Can you work these out from the model? Positions are in its coordinate system, mm. A direction names the side the tool comes from. Round coordinates to 2 decimals unless told otherwise and drop trailing zeros. Loops run counter-clockwise (first coordinate to the right, second up) from the corner with the lowest first, then second, coordinate; pieces in that order, holes last. Notation, with made-up numbers: (50, 14.5) -> (91, 14.5) arc R25 ccw to (91, 27.5) -> close; hole circle Ø4 at (-31.75, 43). An arc over 180 degrees is marked (long way). Use a Markdown table: item, result.
from build123d import *

# Parameters (mm, degrees)
F0_R     = 6
F1_DEPTH = 10


with BuildPart() as f1:
    # F0 (on Top) → F1 (new body)
    with BuildSketch(Plane.XY):
        with BuildLine():
            Line((58.85537, -68.397695), (17.674352, 9.360411))
            ThreePointArc((17.674352, 9.360411), (-7.229789, 18.647524), (-19.364917, -5))
            Line((-19.364917, -5), (0, -80))
            Line((0, -80), (25, -80))
            Line((25, -80), (25, -130))
            Line((25, -130), (56.798395, -90.252006))
            ThreePointArc((56.798395, -90.252006), (61.093013, -79.632266), (58.85537, -68.397695))
        make_face()
        Circle(F0_R, mode=Mode.SUBTRACT)
    extrude(amount=F1_DEPTH)


solid = f1.part
1. I need wall thicknesses on line 1 (X direction, y = -1, z = 2.25); line 2 (X direction, y = -103.5, z = 3); line 3 (X direction, y = -47, z = 0.75). Which ranges of each line are inside material? Lowest first, please.
Answer sheet:
| item | result |
|---|---|
| line 1 | x = -19.97 to -5.92, 5.92 to 23.16 |
| line 2 | x = 25 to 46.2 |
| line 3 | x = -8.52 to 47.52 |
2. I want a section at C-C (x = 39.5). Please give me the cut outline in (y, z) (3 decimals).
Answer sheet:
| item | result |
|---|---|
| outline | (-111.875, 0) -> (-31.851, 0) -> (-31.851, 10) -> (-111.875, 10) -> close |
3. I want a section at D-D (y = -86). Please give me the cut outline in (x, z).
Answer sheet:
| item | result |
|---|---|
| outline | (25, 0) -> (59.4, 0) -> (59.4, 10) -> (25, 10) -> close |
4. If we mould it in two halves opening along X, with no side actions, what happens to faces 1 (the flat face through (12, -80, 5)), 2 (the cylindrical face through (-6, 0, 5)), 3 (the cylindrical face through (61.077, -79.794, 4.93))? For each: +X half, -X half, draft (parallel to the pull), parting line (faces both ways), or undercut.
Answer sheet:
| item | result |
|---|---|
| face 1 | draft |
| face 2 | undercut |
| face 3 | +X half |
5. I want a section at A-A (z = 4). Please give me the cut outline in (x, y), plus the area to 3 significant figures.
Answer sheet:
| item | result |
|---|---|
| outline | (-19.36, -5) -> (0, -80) -> (25, -80) -> (25, -130) -> (56.8, -90.25) arc R20 ccw to (58.86, -68.4) -> (17.67, 9.36) arc R20 ccw to start; hole circle Ø12 at (0, 0) |
| area | 5,820 mm² |
6. Which directions (+Z, -Z, +X, -X, +Y, -Y) give clear straight access to the entire face, cutting with the end or side of a thin tool? Please do faces 4 (the flat face through (41, -110, 5)), 5 (the flat face through (25, -105, 5)).
Answer sheet:
| item | result |
|---|---|
| face 4 | +Z, -Z, +X, -Y |
| face 5 | +Z, -Z, -X, -Y |
7. I want a section at B-B (y = 0). Please give me the cut outline in (x, z).
Answer sheet:
| item | result |
|---|---|
| outline | (-20, 0) -> (-6, 0) -> (-6, 10) -> (-20, 10) -> close; (6, 0) -> (22.63, 0) -> (22.63, 10) -> (6, 10) -> close |
8. Will these pins go through, and if not, where does the flat tip stop? pin 1 Ø3 at (x, z) = (3, 2.5) entering from +Y; pin 2 Ø4 at (y, z) = (4, 3.5) entering from -X; pin 3 Ø6 at (x, z) = (17, 9) entering from -Y.
Answer sheet:
| item | result |
|---|---|
| pin 1 | stops at y = 19.94 |
| pin 2 | stops at x = -19.9 |
| pin 3 | stops at y = -80 |
